Read the model definition and answer for the solid it produces. Units are mm, in the model's axes. Face numbers are marked on the shaded views. A direction names the side the tool comes from. Round coordinates to 2 decimals unless told otherwise and drop trailing zeros. Write each loop counter-clockwise with the first axis right and the second up, starting at its lowest first coordinate (ties: lowest second). Pieces come first, ordered by that corner, then holes. Notation, with made-up numbers: (36, 83) -> (83, 83) arc R4 ccw to (83, 90) -> close; hole circle Ø5 at (47.25, 1). An arc over 180 degrees is marked (long way). Return JSON: item names as keys, results as strings. Group by question number.
(1) For the marked faces 1 and 2, determine the directions among +Z, -Z, +X, -X, +Y, -Y from which every point of the face is accessible in a straight line to the end or side of a thin tool.
(2) A cutting plane is placed at A-A on y = 5.5. Give the vertices of the cut face in (x, z), then the cut area to 3 significant figures.
(3) A cutting plane is placed at D-D on x = -1.5. Give the vertices of the cut face in (y, z).
(4) Straight lines are drawn through the part: line 1 (Y direction, x = 16, z = -0.75); line 2 (X direction, y = 33, z = -7); line 3 (Y direction, x = 13.5, z = 0.75). For each, find the intervals that lie inside material, in ascending order.
(5) The mould has two halves that part along X. Classify the marked faces 3, 4 and 5: released by +X, released by -X, zero draft, split by the parting line, or undercut.
(6) Given pin 1 (1.5 mm diameter, centred on x = 3.5, y = -3, fed in from +Z); pin 2 (5 mm diameter, centred on x = -12.5, z = -10, fed in from +Y); pin 3 (10 mm diameter, centred on x = -2.5, z = 5, fed in from -Y); pin 4 (12.5 mm diameter, centred on x = -2.5, z = -5.5, fed in from +Y), each flat-ended and moving along its own axis, determine where each tip first touches the part or whether it passes through.
(7) A cutting plane is placed at C-C on x = -12. Give the vertices of the cut face in (y, z).
```python
from build123d import *

# Parameters (mm, degrees)
BASE_EXTRUDE_DEPTH = 12.7


with BuildPart() as part:
    # Sketch1 → Base-Extrude (new, symmetric)
    with BuildSketch(Plane.XY):
        with BuildLine():
            Line((-20.6375, 36.5125), (-20.6375, 2.6924))
            ThreePointArc((-20.6375, 2.6924), (-19.848914298, 0.788585702), (-17.9451, 0))
            Line((-17.9451, 0), (17.9451, 0))
            ThreePointArc((17.9451, 0), (19.848914298, 0.788585702), (20.6375, 2.6924))
            Line((20.6375, 2.6924), (20.6375, 36.5125))
            ThreePointArc((20.6375, 36.5125), (15.875, 41.275), (11.1125, 36.5125))
            Line((11.1125, 36.5125), (11.1125, 35.47745))
            ThreePointArc((11.1125, 35.47745), (12.4587, 34.13125), (13.8049, 35.47745))
            Line((13.8049, 35.47745), (13.8049, 36.5125))
            ThreePointArc((13.8049, 36.5125), (15.875, 38.5826), (17.9451, 36.5125))
            Line((17.9451, 36.5125), (17.9451, 2.6924))
            Line((17.9451, 2.6924), (-17.9451, 2.6924))
            Line((-17.9451, 2.6924), (-17.9451, 36.5125))
            ThreePointArc((-17.9451, 36.5125), (-15.875, 38.5826), (-13.8049, 36.5125))
            Line((-13.8049, 36.5125), (-13.8049, 35.47745))
            ThreePointArc((-13.8049, 35.47745), (-12.4587, 34.13125), (-11.1125, 35.47745))
            Line((-11.1125, 35.47745), (-11.1125, 36.5125))
            ThreePointArc((-11.1125, 36.5125), (-15.875, 41.275), (-20.6375, 36.5125))
        make_face()
    base_extrude = extrude(amount=BASE_EXTRUDE_DEPTH, both=True)

    # Mirror1: Base-Extrude across plane
    add(base_extrude.mirror(Plane.ZX))


solid = part.part
```
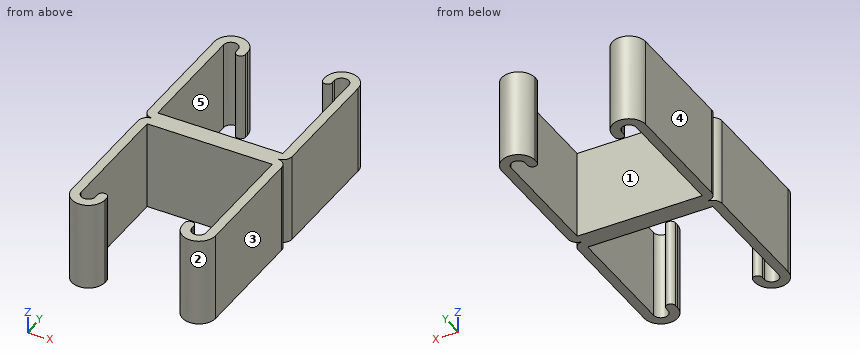
Checks:
{
 "1": {"face 1": "+Z, -Z", "face 2": "+Z, -Z, -Y"},
 "2": {"outline": "(-20.64, -12.7) -> (-17.95, -12.7) -> (-17.95, 12.7) -> (-20.64, 12.7) -> close; (17.95, -12.7) -> (20.64, -12.7) -> (20.64, 12.7) -> (17.95, 12.7) -> close", "area": "137 mm^2"},
 "3": {"outline": "(-2.69, -12.7) -> (2.69, -12.7) -> (2.69, 12.7) -> (-2.69, 12.7) -> close"},
 "4": {"line 1": "y = -41.27 to -38.58, -2.69 to 2.69, 38.58 to 41.27", "line 2": "x = -20.64 to -17.95, 17.95 to 20.64", "line 3": "y = -40.64 to -34.62, -2.69 to 2.69, 34.62 to 40.64"},
 "5": {"face 3": "released by +X", "face 4": "released by -X", "face 5": "undercut"},
 "6": {"pin 1": "stops at z = 12.7", "pin 2": "stops at y = 41.19", "pin 3": "stops at y = -2.69", "pin 4": "stops at y = 2.69"},
 "7": {"outline": "(-39.28, -12.7) -> (-34.21, -12.7) -> (-34.21, 12.7) -> (-39.28, 12.7) -> close; (-2.69, -12.7) -> (2.69, -12.7) -> (2.69, 12.7) -> (-2.69, 12.7) -> close; (34.21, -12.7) -> (39.28, -12.7) -> (39.28, 12.7) -> (34.21, 12.7) -> close"}
}
